Here's how the part is built. I have some questions about the finished solid (model axes, mm). Give positions to 0.01 mm unless a question says otherwise; leave off trailing zeros. Write each loop counter-clockwise with the first axis right and the second up, starting at its lowest first coordinate (ties: lowest second). Pieces come first, ordered by that corner, then holes. Notation, with made-up numbers: (50.25, 44.5) -> (82.25, 44.5) arc R29 cw to (82.25, 68.5) -> close; hole circle Ø1 at (-6, 29.5). An arc over 180 degrees is marked (long way). Use CSV: the item, a comma, the result in double quotes. Start each with the question number.
(1) Suppose I cut it at C-C on y = 0. List the corners of the cut face in (x, z) for me.
(2) Suppose I cut it at B-B on x = 2.5. List the corners of the cut face in (y, z) for me, plus the area to 3 significant figures.
(3) For pin 1 Ø4 at (y, z) = (3, 1.5) entering from -X; pin 2 Ø3 at (y, z) = (-2, 1.5) entering from +X; pin 3 Ø4 at (y, z) = (6, 0.5) entering from -X, each with a flat end and sliding along its axis, tell me the tip position at first contact or that it passes through.
(4) If we mould it in two halves opening along X, with no side actions, what happens to faces 1 (the flat face through (-2, 4, 4.5)), 2 (the cylindrical face through (0.867, -3.905, -0.063)), 3 (the flat face through (3.82, 5.79, 0.06)), 4 (the flat face through (-3.82, -5.79, 0.06))? For each: pulls with the +X half, pulls with the -X half, needs draft (parallel to the pull), parting line crosses it, or undercut.
(5) I need wall thicknesses on L1, parallel to Y at x = 0, z = -1; L2, parallel to X at y = 2, z = 1; L3, parallel to X at y = 3.5, z = 3. Which ranges of each line are inside material? Lowest first, please. Write a range as [from, to].
(6) Suppose I cut it at D-D on x = 5.75. List the corners of the cut face in (y, z) for me.
(7) Suppose I cut it at A-A on z = 3.75. List the corners of the cut face in (x, y) for me.
from build123d import *

# Parameters (mm, degrees)
BOSS_EXTRUDE1_DEPTH = 4.5
SKETCH2_R           = 4
CUT_EXTRUDE1_DEPTH  = 9


with BuildPart() as part:
    # Sketch1 → Boss-Extrude1 (new body, symmetric)
    with BuildSketch(Plane.XY):
        Polygon((6.723407542, -4.354716537), (7.132998919, 3.645283463), (0.409591377, 8), (-6.723407542, 4.354716537), (-7.132998919, -3.645283463), (-0.409591377, -8), align=None)
    extrude(amount=BOSS_EXTRUDE1_DEPTH, both=True)

    # Sketch2 → Cut-Extrude1 (cut)
    with BuildSketch(Plane(origin=(0, 0, -4.5), x_dir=(-1, 0, 0), z_dir=(0, 0, -1))):
        Circle(SKETCH2_R)
    extrude(amount=-CUT_EXTRUDE1_DEPTH, mode=Mode.SUBTRACT)


solid = part.part
Geometry says:
1,outline,"(-6.95, -4.5) -> (-4, -4.5) -> (-4, 4.5) -> (-6.95, 4.5) -> close; (4, -4.5) -> (6.95, -4.5) -> (6.95, 4.5) -> (4, 4.5) -> close"
2,outline,"(-6.51, -4.5) -> (-3.12, -4.5) -> (-3.12, 4.5) -> (-6.51, 4.5) -> close; (3.12, -4.5) -> (6.65, -4.5) -> (6.65, 4.5) -> (3.12, 4.5) -> close"
2,area,"62.2 mm²"
3,pin 1,"x = -6.9"
3,pin 2,"x = 6.92"
3,pin 3,"x = -6.74"
4,face 1,"needs draft"
4,face 2,"undercut"
4,face 3,"pulls with the +X half"
4,face 4,"pulls with the -X half"
5,L1,"[-7.79, -4], [4, 7.79]"
5,L2,"[-6.84, -3.46], [3.46, 7.05]"
5,L3,"[-6.77, -1.94], [1.94, 7.13]"
6,outline,"(-4.85, -4.5) -> (4.54, -4.5) -> (4.54, 4.5) -> (-4.85, 4.5) -> close"
7,outline,"(-7.13, -3.65) -> (-0.41, -8) -> (6.72, -4.35) -> (7.13, 3.65) -> (0.41, 8) -> (-6.72, 4.35) -> close; hole circle Ø8 at (0, 0)"
